Work out the finished part from the listing and answer in its coordinate system (mm). Face numbers are marked on the shaded views. A direction names the side the tool comes from. Give positions to 0.01 mm unless a question says otherwise; leave off trailing zeros. Loops run counter-clockwise (first coordinate to the right, second up) from the corner with the lowest first, then second, coordinate; pieces in that order, holes last. Notation, with made-up numbers: (-34.5, 20.5) -> (2.5, 20.5) arc R33 cw to (2.5, 53.5) -> close; hole circle Ø1 at (-38, 26.5). An arc over 180 degrees is marked (long way). Answer as CSV lines item,"result". Start each with the question number.
1. Find section A-A, the plane z = 2.25. Give the vertices of the cut face in (x, y).
2. Find section D-D, the plane x = -42. Give the vertices of the cut face in (y, z), and give its area (3 significant figures).
3. Find section C-C, the plane y = 0. Give the vertices of the cut face in (x, z).
4. Flat-ended cylindrical pins translate along their axes: pin 1 Ø9.5 at (x, z) = (-31, 10.5) entering from -Y; pin 2 Ø3 at (x, y) = (-68, 3.5) entering from +Z; pin 3 Ø4 at (x, y) = (-22, -9) entering from +Z. Find the tip coordinate at first contact, or state that the pin passes through.
5. Find the intervals of material crossed by line 1 along X through (y, z) = (3.25, -5.5); line 2 along X through (y, z) = (-0.5, 0.25); line 3 along Y through (x, z) = (-40, -7), in increasing order.
6. Determine the mould class of the marked faces 4, 5, 6 and 7 for opening direction Y: +Y half, -Y half, draft (parallel to the pull), parting line (faces both ways), or undercut.
7. A tool of negligible diameter and unlimited length cuts with its end or side. For the marked faces 1, 2 and 3, from which of +Z, -Z, +X, -X, +Y, -Y can it reach the whole face along a straight path? Write none if from no direction.
8. Find section B-B, the plane x = -50.5. Give the vertices of the cut face in (y, z), and give its area (3 significant figures).
from build123d import *

# Parameters (mm, degrees)
F0_W     = 25.4
F0_H     = 25.4
F1_DEPTH = 76.2
F2_W     = 6.35
F2_H     = 8.636
F3_DEPTH = 76.2
F4_R     = 5.08
F5_DEPTH = 19.05
F6_R     = 5.5499
F7_DEPTH = 73.406


with BuildPart() as f1:
    # F0 (on Right) → F1 (new body)
    with BuildSketch(Plane.YZ):
        Rectangle(F0_W, F0_H)
    extrude(amount=-F1_DEPTH)

    # F2 (on Right) → F3 (cut)
    with BuildSketch(Plane.YZ):
        with Locations((-9.525, 8.382)):
            Rectangle(F2_W, F2_H)
    extrude(amount=-F3_DEPTH, mode=Mode.SUBTRACT)

    # F4 (on face) → F5 (cut)
    with BuildSketch(Plane.XY.offset(12.7)):
        with Locations((-66.294, 3.048)):
            Circle(F4_R)
        with Locations((-9.906, 3.048)):
            Circle(F4_R)
    extrude(amount=-F5_DEPTH, mode=Mode.SUBTRACT)

    # F6 (on face) → F7 (cut)
    with BuildSketch(Plane.XY.offset(12.7)):
        with Locations((-39.878, 3.048)):
            Circle(F6_R)
    extrude(amount=-F7_DEPTH, mode=Mode.SUBTRACT)


solid = f1.part
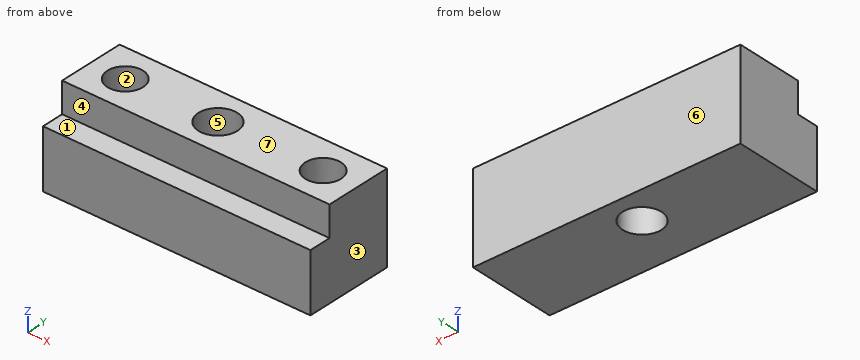
Resolved:
1,outline,"(-76.2, -12.7) -> (0, -12.7) -> (0, 12.7) -> (-76.2, 12.7) -> close; hole circle Ø10.16 at (-66.29, 3.05); hole circle Ø11.1 at (-39.88, 3.05); hole circle Ø10.16 at (-9.91, 3.05)"
2,outline,"(-12.7, -12.7) -> (-2.08, -12.7) -> (-2.08, 12.7) -> (-6.35, 12.7) -> (-6.35, 4.06) -> (-12.7, 4.06) -> close; (8.18, -12.7) -> (12.7, -12.7) -> (12.7, 12.7) -> (8.18, 12.7) -> close"
2,area,"330 mm^2"
3,outline,"(-76.2, -12.7) -> (-44.52, -12.7) -> (-44.52, 12.7) -> (-62.23, 12.7) -> (-62.23, -6.35) -> (-70.36, -6.35) -> (-70.36, 12.7) -> (-76.2, 12.7) -> close; (-35.24, -12.7) -> (0, -12.7) -> (0, 12.7) -> (-5.84, 12.7) -> (-5.84, -6.35) -> (-13.97, -6.35) -> (-13.97, 12.7) -> (-35.24, 12.7) -> close"
4,pin 1,"stops at y = -6.35"
4,pin 2,"stops at z = -6.35"
4,pin 3,"stops at z = 4.06"
5,line 1,"x = -76.2 to -71.37, -61.22 to -45.42, -34.33 to -14.98, -4.83 to 0"
5,line 2,"x = -76.2 to -69.93, -62.66 to -44.15, -35.61 to -13.54, -6.27 to 0"
5,line 3,"y = -12.7 to -2.5, 8.6 to 12.7"
6,face 4,"-Y half"
6,face 5,"undercut"
6,face 6,"+Y half"
6,face 7,"draft"
7,face 1,"+Z, +X, -X, -Y"
7,face 2,"+Z"
7,face 3,"+Z, -Z, +X, +Y, -Y"
8,outline,"(-12.7, -12.7) -> (12.7, -12.7) -> (12.7, 12.7) -> (-6.35, 12.7) -> (-6.35, 4.06) -> (-12.7, 4.06) -> close"
8,area,"590 mm^2"
